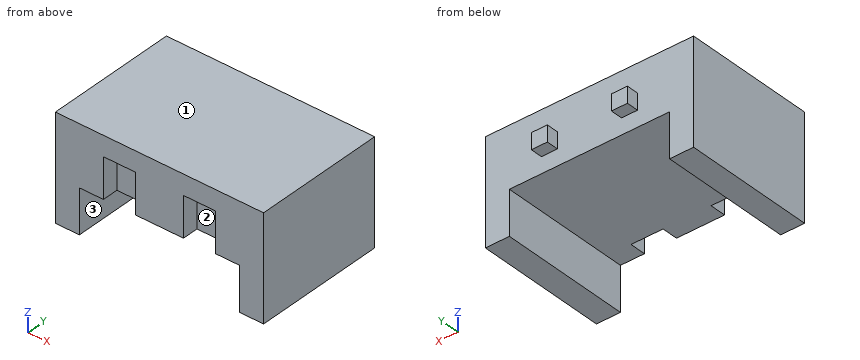
from build123d import *

# Parameters (mm, degrees)
EXTRUDE_1_DEPTH     = 16.5
SKETCH_2_W          = 4
SKETCH_2_H          = 5
CUT_EXTRUDE_1_DEPTH = 2
SKETCH_3_W          = 2
SKETCH_3_H          = 2
EXTRUDE_2_DEPTH     = 1.5


with BuildPart() as part:
    # Эскиз1 → Бобышка-Вытянуть1 (new body)
    with BuildSketch(Plane(origin=(0, 0, 0), x_dir=(1, 0, 0), z_dir=(0, 1, 0))):
        Polygon((-10, 1), (10, 1), (10, 6.5), (13, 6.5), (13, -6.5), (-13, -6.5), (-13, 6.5), (-10, 6.5), align=None)
    extrude(amount=EXTRUDE_1_DEPTH)

    # Эскиз2 → Вырез-Вытянуть1 (cut)
    with BuildSketch(Plane(origin=(0, 0, 0), x_dir=(-1, 0, 0), z_dir=(0, -1, 0))):
        with Locations((-5, -1.5)):
            Rectangle(SKETCH_2_W, SKETCH_2_H)
        with Locations((5, -1.5)):
            Rectangle(SKETCH_2_W, SKETCH_2_H)
    extrude(amount=-CUT_EXTRUDE_1_DEPTH, mode=Mode.SUBTRACT)

    # Эскиз3 → Бобышка-Вытянуть2 (add)
    with BuildSketch(Plane(origin=(0, 16.5, 0), x_dir=(1, 0, 0), z_dir=(0, 1, 0))):
        with Locations((-5, -2)):
            Rectangle(SKETCH_3_W, SKETCH_3_H)
        with Locations((5, -2)):
            Rectangle(SKETCH_3_W, SKETCH_3_H)
    extrude(amount=EXTRUDE_2_DEPTH)


solid = part.part
For this review, take the finished solid that the model builds, in its own axes (mm). Face numbers are marked on the shaded views. A direction names the side the tool comes from. Round coordinates to 2 decimals unless told otherwise and drop trailing zeros. Order: outer loops, then holes, each group sorted by start corner. A loop starts at its lowest first (then second) coordinate and runs counter-clockwise, first axis right, second up. Notation, with made-up numbers: M -30.75,-35 L -7.75,-35 A35 cw -7.75,-2 Z; hole C -34,27.5 d10. An arc over 180 degrees is marked long. Use a Markdown table: item, result. Add a question column.
Item 1: Add section D-D, the plane z = 0.5. Give the boundary of the cut face in (x, y).
Item 2: Add section A-A, the plane z = -5.5. Give the boundary of the cut face in (x, y).
Item 3: Insertion check: pin 1 (0.8 mm diameter, centred on x = 5, y = 17.5, fed in from -Z); pin 2 (1.6 mm diameter, centred on y = 17.5, z = 2, fed in from -X); pin 3 (2 mm diameter, centred on x = 6, y = 1.5, fed in from -Z). Each pin has a flat end and moves straight along its axis. Give the tip position at first contact, or say it passes through.
Item 4: Add section C-C, the plane x = 5.25. Give the boundary of the cut face in (y, z).
Item 5: Add section B-B, the plane y = 7.5. Give the boundary of the cut face in (x, z).
Item 6: Tool access review of the marked faces 1, 2 and 3: name each direction out of +Z, -Z, +X, -X, +Y, -Y from which nothing blocks a thin tool from reaching the whole face with its end or side.
Item 7: To check wall thickness, follow line 1 along X through (y, z) = (1.5, 3.5); line 2 along X through (y, z) = (12.5, -1.25); line 3 along Y through (x, z) = (11, -1). State the ranges of each line that lie inside material, in increasing order.
Geometry results:
| question | item | result |
|---|---|---|
| 1 | outline | M -13,0 L -7,0 L -7,2 L -3,2 L -3,0 L 3,0 L 3,2 L 7,2 L 7,0 L 13,0 L 13,16.5 L -13,16.5 Z |
| 2 | outline | M -13,0 L -10,0 L -10,16.5 L -13,16.5 Z; M 10,0 L 13,0 L 13,16.5 L 10,16.5 Z |
| 3 | pin 1 | stops at z = 1 |
| 3 | pin 2 | stops at x = -6 |
| 3 | pin 3 | stops at z = -1 |
| 4 | outline | M 0,4 L 2,4 L 2,-1 L 16.5,-1 L 16.5,1 L 18,1 L 18,3 L 16.5,3 L 16.5,6.5 L 0,6.5 Z |
| 5 | outline | M -13,-6.5 L -10,-6.5 L -10,-1 L 10,-1 L 10,-6.5 L 13,-6.5 L 13,6.5 L -13,6.5 Z |
| 6 | face 1 | +Z, +X, -X, +Y, -Y |
| 6 | face 2 | -Z, -Y |
| 6 | face 3 | -Z, +Y, -Y |
| 7 | line 1 | x = -13 to -7, -3 to 3, 7 to 13 |
| 7 | line 2 | x = -13 to -10, 10 to 13 |
| 7 | line 3 | y = 0 to 16.5 |
